Can you work these out from the model? Positions are in its coordinate system, mm. Face numbers are marked on the shaded views. Round coordinates to 2 decimals unless told otherwise and drop trailing zeros. Loops run counter-clockwise (first coordinate to the right, second up) from the corner with the lowest first, then second, coordinate; pieces in that order, holes last. Notation, with made-up numbers: M -19,-33.5 L 28,-33.5 A20 ccw 28,-27.5 Z; hole C 54.25,29.25 d2. An arc over 180 degrees is marked long. Answer as CSV lines item,"result".
Autodesk Inventor part; units mm, degrees
ref_plane "YZ Plane" through (0, 0, 0) normal (1, 0, 0) x (0, 1, 0)
ref_plane "XZ Plane" through (0, 0, 0) normal (0, 1, 0) x (-1, 0, 0)
ref_plane "XY Plane" through (0, 0, 0) normal (0, 0, 1) x (1, 0, 0)
sketch "Sketch1" plane through (0, 0, 0) normal (0, 0, 1) x (1, 0, 0)
  line L0 (-15.8764, 0) -> (-29.8764, 0)
  line L1 (-15.8764, 0) -> (-7.3764, 0)
  line L2 (-25.9706, 16.9706) -> (-25.9706, -16.9706) construction
  line L3 (-7.9706, -16.9706) -> (-7.9706, 16.9706) construction
  arc A0 (-7.9706, 16.9706) -> (-7.9926, 17.6) centre (-16.9706, 16.9706) ccw construction
  arc A1 (-25.9706, -16.9706) -> (-25.0651, -20.9049) centre (-16.9706, -16.9706) ccw construction
  arc A2 (-25.0651, 20.9049) -> (-25.0651, -20.9049) centre (17.9444, 0) ccw
  arc A3 (-7.9926, -17.6) -> (-7.9926, 17.6) centre (-259.0334, 0) ccw
  arc A4 (-25.0651, 20.9049) -> (-25.9706, 16.9706) centre (-16.9706, 16.9706) ccw construction
  arc A5 (-25.0651, -20.9049) -> (-7.9926, -17.6) centre (-16.9706, -16.9706) ccw
  arc A6 (-7.9926, 17.6) -> (-25.0651, 20.9049) centre (-16.9706, 16.9706) ccw
  arc A7 (-7.9926, -17.6) -> (-7.9706, -16.9706) centre (-16.9706, -16.9706) ccw construction
  line L4 (-16.9706, -20.5501) -> (-20.0706, -15.1808) construction
  line L5 (-20.0706, -15.1808) -> (-13.8706, -15.1808) construction
  line L6 (-13.8706, -15.1808) -> (-16.9706, -20.5501) construction
  circle A8 centre (-20.0706, -15.1808) radius 1.25
  circle A9 centre (-13.8706, -15.1808) radius 1.25
  circle A10 centre (-16.9706, -20.5501) radius 1.25
  line L7 (0, 0) -> (-43.2466, 0) construction
  line L8 (-15.1808, 20.0706) -> (-15.1808, 13.8706) construction
  line L9 (-15.1808, 13.8706) -> (-20.5501, 16.9706) construction
  line L10 (-20.5501, 16.9706) -> (-15.1808, 20.0706) construction
  circle A11 centre (-15.1808, 13.8706) radius 1.25
  circle A12 centre (-20.5501, 16.9706) radius 1.25
  circle A13 centre (-15.1808, 20.0706) radius 1.25
  line L11 (-16.9706, 16.9706) -> (0, 0) construction
  line L12 (-16.9706, -16.9706) -> (0, 0) construction
  point P0 (-29.8764, 0)
  point P1 (-7.3764, 0)
  dimension "d11" = 9
  dimension "d14" = 2.5
  dimension "d15" = 2.5
  dimension "d16" = 2.5
  dimension "d17" = 6.2
  dimension "d19" = 2.5
  dimension "d20" = 2.5
  dimension "d21" = 2.5
  dimension "d22" = 6.2
  dimension "d23" = 24
  dimension "d24" = 45
  dimension "d25" = 24
  dimension "d26" = 45
  dimension "d27" = 14
  dimension "d28" = 8.5
extrude "Extrusion1" add sketch "Sketch1" along normal blind 3
sketch "Sketch2" plane through (0, 0, 3) normal (0, 0, 1) x (1, 0, 0)
  arc A0 (-25.0651, 20.9049) -> (-25.0651, -20.9049) centre (17.9444, 0) ccw
  arc A1 (-25.0651, -20.9049) -> (-7.9926, -17.6) centre (-16.9706, -16.9706) ccw
  arc A2 (-7.9926, -17.6) -> (-7.9926, 17.6) centre (-259.0334, 0) ccw
  arc A3 (-7.9926, 17.6) -> (-25.0651, 20.9049) centre (-16.9706, 16.9706) ccw
  circle A4 centre (-16.9706, -20.5501) radius 1.25
  circle A5 centre (-13.8706, -15.1808) radius 1.25
  circle A6 centre (-20.0706, -15.1808) radius 1.25
  circle A7 centre (-15.1808, 13.8706) radius 1.25
  circle A8 centre (-15.1808, 20.0706) radius 1.25
  circle A9 centre (-20.5501, 16.9706) radius 1.25
  arc A10 (-23.2663, 20.0306) -> (-23.2663, -20.0306) centre (17.9444, 0) ccw
  arc A11 (-9.9877, 17.4601) -> (-23.2663, 20.0306) centre (-16.9706, 16.9706) ccw
  arc A12 (-9.9877, -17.4601) -> (-9.9877, 17.4601) centre (-259.0334, 0) ccw
  arc A13 (-23.2663, -20.0306) -> (-9.9877, -17.4601) centre (-16.9706, -16.9706) ccw
  circle A14 centre (-15.1808, 13.8706) radius 4.25
  circle A15 centre (-16.9706, 16.9706) radius 7.8296
  circle A16 centre (-16.9706, -16.9706) radius 7.8296
  line L0 (-9.7642, 13.9095) -> (10.6825, 13.9095)
  point P0 (0, 0)
  point P1 (-24.7881, -16.5371)
  point P2 (-9.7642, -13.9095)
  point P3 (-24.7881, 16.5371)
  dimension "d33" = 15.6591
  dimension "d31" = 2
  dimension "d32" = 3
  dimension "d34" = 15.6591
extrude "Extrusion2" cut sketch "Sketch2" against normal blind 2 contours A15 A12 A16 A10
fillet "Fillet1" radius 7 2 edges at (-24.7881, 16.5371, 2) (-9.7642, -13.9095, 2)
fillet "Fillet2" radius 2 2 edges at (-9.7642, 13.9095, 2) (-24.7881, -16.5371, 2)
sketch "Sketch3" plane through (0, 0, 3) normal (0, 0, 1) x (1, 0, 0)
  arc A0 (-18.9853, 9.4046) -> (-12.6387, 10.4485) centre (-16.9706, 16.9706) ccw
  arc A1 (-9.5334, 8.8534) -> (-12.6387, 10.4485) centre (-11.5322, 8.7825) ccw
  arc A2 (-9.3862, -2.2146) -> (-9.5334, 8.8534) centre (-259.0334, 0) ccw
  arc A3 (-16.6619, -9.1471) -> (-9.3862, -2.2146) centre (-16.386, -2.1525) ccw
  arc A4 (-16.6619, -9.1471) -> (-23.006, -11.983) centre (-16.9706, -16.9706) ccw
  arc A5 (-26.4871, -11.1978) -> (-23.006, -11.983) centre (-24.5477, -10.709) ccw
  arc A6 (-27.7703, 3.1165) -> (-26.4871, -11.1978) centre (17.9444, 0) ccw
  arc A7 (-18.9853, 9.4046) -> (-27.7703, 3.1165) centre (-20.7865, 2.6404) ccw
  arc A8 (-25.0651, 20.9049) -> (-25.0651, -20.9049) centre (17.9444, 0) ccw
  arc A9 (-25.0651, -20.9049) -> (-7.9926, -17.6) centre (-16.9706, -16.9706) ccw
  arc A10 (-7.9926, -17.6) -> (-7.9926, 17.6) centre (-259.0334, 0) ccw
  arc A11 (-7.9926, 17.6) -> (-25.0651, 20.9049) centre (-16.9706, 16.9706) ccw
  circle A12 centre (-16.9706, -20.5501) radius 1.25
  circle A13 centre (-13.8706, -15.1808) radius 1.25
  circle A14 centre (-20.0706, -15.1808) radius 1.25
  circle A15 centre (-15.1808, 13.8706) radius 1.25
  circle A16 centre (-15.1808, 20.0706) radius 1.25
  circle A17 centre (-20.5501, 16.9706) radius 1.25
  point P0 (0, 0)
equation "\"d34\" = d33"
properties part number "クランク"
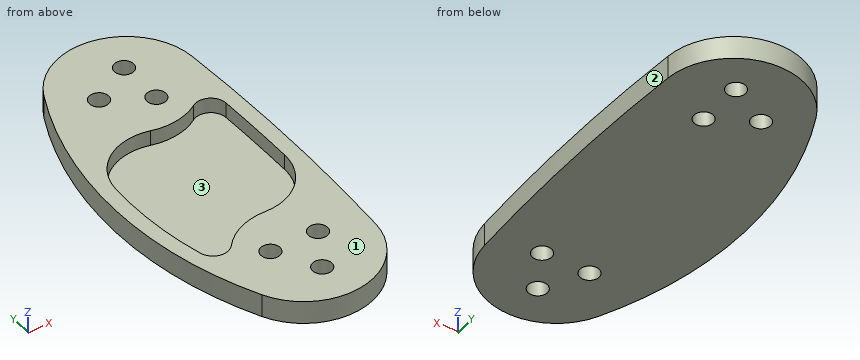
Item 1: If we section it at B-B on x = -14.5: State how many separate pieces and enclosed holes the cut face has, then the cut area to 3 significant figures.
Output:
separate pieces,"4"
enclosed holes,"0"
area,"97.8 mm2"
Item 2: If I drill on line 1 along Y through (x, z) = (-19.5, 1.6); line 2 along Y through (x, z) = (-17.5, 1.05) (3 decimals); line 3 along X through (y, z) = (-15, 2.55), over which ranges is the centre line in solid material (lowest first)? Write a range as from..to.
Output:
line 1,"y = -25.61..-16.29, -14.07..-9.56, 9.52..16.29, 17.65..25.61"
line 2,"y = -25.955..-21.682, -19.418..-9.159, 9.159..25.955"
line 3,"x = -27.46..-21.31, -18.83..-15.11, -12.63..-7.82"
Item 3: Will these pins go through, and if not, where does the flat tip stop? pin 1 (2 mm diameter, centred on x = -27.5, y = 17, fed in from +Z); pin 2 (2 mm diameter, centred on x = -20.55, y = 16.97, fed in from +Z); pin 3 (1 mm diameter, centred on x = -18.5, z = 1.5, fed in from +Y); pin 4 (1.5 mm diameter, centred on x = -14, z = 2.5, fed in from +Y).
Output:
pin 1,"stops at z = 3"
pin 2,"passes through"
pin 3,"stops at y = 25.91"
pin 4,"stops at y = 25.69"
Item 4: We'd pull the mould along Y, two halves only. Please class the marked faces 1, 2 and 3: released by +Y, released by -Y, zero draft, split by the parting line, or undercut.
Output:
face 1,"zero draft"
face 2,"split by the parting line"
face 3,"undercut"
Item 5: If we section it at A-A on y = 0: Write out the boundary of the cut face in (x, z).
Output:
outline,"M -29.88,0 L -7.38,0 L -7.38,3 L -9.38,3 L -9.38,1 L -27.88,1 L -27.88,3 L -29.88,3 Z"
